Here's the drawing with two shaded views (mm, measured from the low corner). I have some questions. Coordinates: 2 decimals unless noted, no trailing zeros. Loops run counter-clockwise (first coordinate to the right, second up) from the corner with the lowest first, then second, coordinate; pieces in that order, holes last. Notation, with made-up numbers: (49.5, 44.25) -> (70.5, 44.25) arc R13 ccw to (70.5, 65.25) -> close; hole circle Ø11 at (-8.5, -14.75). An arc over 180 degrees is marked (long way). Answer as a JSON object with one key per item and string values. Group by question number.
1) I want a section at C-C (y = 16). Write out the boundary of the cut face in (x, z), then the cut area to 3 significant figures.
2) I need wall thicknesses on probe 1 along X at (y, z) = (0.4, 5); probe 2 along Z at (x, y) = (6, 0.5); probe 3 along Y at (x, z) = (1.1, 15). Which ranges of each line are inside material? Lowest first, please. Write a range as [from, to].
3) If we mould it in two halves opening along X, with no side actions, what happens to the marked faces 1, 2 and 3? For each: +X half, -X half, draft (parallel to the pull), parting line (faces both ways), or undercut.
4) I want a section at B-B (z = 5). Write out the boundary of the cut face in (x, y).
5) I want a section at D-D (z = 15). Write out the boundary of the cut face in (x, y).
6) I'm going to push flat-ended pins straight in: pin 1 (3 mm diameter, centred on y = 4, z = 19.5, fed in from -X); pin 2 (8.5 mm diameter, centred on y = 9, z = 9, fed in from +X); pin 3 (1.5 mm diameter, centred on x = 8.5, z = 22.5, fed in from +Y). Where does each tip first touch, or does it pass through?
7) I want a section at A-A (x = 16). Write out the boundary of the cut face in (y, z).
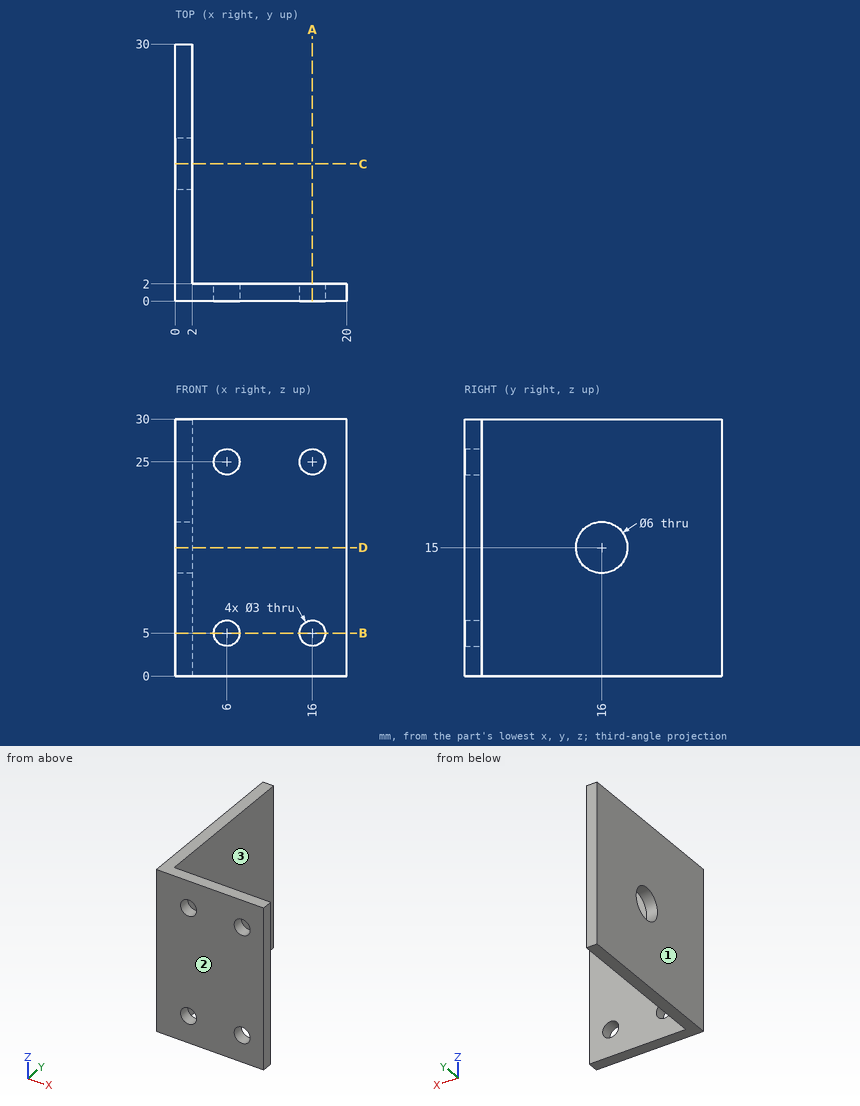
Determined:
{
 "1": {"outline": "(0, 0) -> (2, 0) -> (2, 12) -> (0, 12) -> close; (0, 18) -> (2, 18) -> (2, 30) -> (0, 30) -> close", "area": "48.0 mm^2"},
 "2": {"probe 1": "[0, 4.5], [7.5, 14.5], [17.5, 20]", "probe 2": "[0, 3.5], [6.5, 23.5], [26.5, 30]", "probe 3": "[0, 13], [19, 30]"},
 "3": {"face 1": "-X half", "face 2": "draft", "face 3": "+X half"},
 "4": {"outline": "(0, 0) -> (4.5, 0) -> (4.5, 2) -> (2, 2) -> (2, 30) -> (0, 30) -> close; (7.5, 0) -> (14.5, 0) -> (14.5, 2) -> (7.5, 2) -> close; (17.5, 0) -> (20, 0) -> (20, 2) -> (17.5, 2) -> close"},
 "5": {"outline": "(0, 0) -> (20, 0) -> (20, 2) -> (2, 2) -> (2, 13) -> (0, 13) -> close; (0, 19) -> (2, 19) -> (2, 30) -> (0, 30) -> close"},
 "6": {"pin 1": "x = 0", "pin 2": "x = 2", "pin 3": "y = 2"},
 "7": {"outline": "(0, 0) -> (2, 0) -> (2, 3.5) -> (0, 3.5) -> close; (0, 6.5) -> (2, 6.5) -> (2, 23.5) -> (0, 23.5) -> close; (0, 26.5) -> (2, 26.5) -> (2, 30) -> (0, 30) -> close"}
}
